Geometry check sheet. Reference: the model listing, model coordinates, mm. A direction names the side the tool comes from. Coordinates: 2 decimals unless noted, no trailing zeros. Write each loop counter-clockwise with the first axis right and the second up, starting at its lowest first coordinate (ties: lowest second). Pieces come first, ordered by that corner, then holes.
from build123d import *

# Parameters (mm, degrees)
SKETCH1_W                      = 65
SKETCH1_H                      = 100
BOSS_EXTRUDE1_DEPTH            = 5
SKETCH2_R                      = 3.5
BOSS_EXTRUDE2_DEPTH            = 3
F_3_6_3_6_DIAMETER_HOLE1_D     = 3.6
CBORE_FOR_M3_SHCS1_D           = 3.4
CBORE_FOR_M3_SHCS1_CBORE_D     = 6.5
CBORE_FOR_M3_SHCS1_CBORE_DEPTH = 3
SKETCH9_W                      = 100
SKETCH9_H                      = 5
BOSS_EXTRUDE3_DEPTH            = 50
CBORE_FOR_M3_SHCS2_D           = 3.4
CBORE_FOR_M3_SHCS2_CBORE_D     = 6.5
CBORE_FOR_M3_SHCS2_CBORE_DEPTH = 3
F_5_1_5_1_DIAMETER_HOLE1_D     = 5.1
CUT_EXTRUDE1_DEPTH             = 1
FILLET1_R                      = 1
FILLET2_R                      = 5
CHAMFER2_SIZE                  = 0.5


with BuildPart() as part:
    # Sketch1 → Boss-Extrude1 (new body)
    with BuildSketch(Plane(origin=(0, 0, 0), x_dir=(1, 0, 0), z_dir=(0, 1, 0))):
        with Locations((32.5, -50)):
            Rectangle(SKETCH1_W, SKETCH1_H)
    extrude(amount=BOSS_EXTRUDE1_DEPTH)

    # Sketch2 → Boss-Extrude2 (add)
    with BuildSketch(Plane(origin=(0, 5, 0), x_dir=(1, 0, 0), z_dir=(0, 1, 0))):
        with Locations(Location((8, -21, 0), (0, 0, 270))):
            Circle(SKETCH2_R)
        with Locations(Location((57, -21, 0), (0, 0, 270))):
            Circle(SKETCH2_R)
        with Locations(Location((57, -79, 0), (0, 0, 270))):
            Circle(SKETCH2_R)
        with Locations(Location((8, -79, 0), (0, 0, 270))):
            Circle(SKETCH2_R)
    extrude(amount=BOSS_EXTRUDE2_DEPTH)

    # Ø3.6 (3.6) Diameter Hole1 (through all)
    with Locations(Plane(origin=(0, 8, 0), x_dir=(1, 0, 0), z_dir=(0, 1, 0))):
        with Locations((8, -21), (57, -21), (57, -79), (8, -79)):
            Hole(F_3_6_3_6_DIAMETER_HOLE1_D / 2)

    # CBORE for M3 SHCS1 (through all)
    with Locations(Plane(origin=(0, 5, 0), x_dir=(1, 0, 0), z_dir=(0, 1, 0))):
        with Locations((17.5, -7.5), (47.5, -7.5)):
            CounterBoreHole(CBORE_FOR_M3_SHCS1_D / 2, CBORE_FOR_M3_SHCS1_CBORE_D / 2, CBORE_FOR_M3_SHCS1_CBORE_DEPTH)

    # Sketch9 → Boss-Extrude3 (add)
    with BuildSketch(Plane.ZY):
        with Locations((50, 2.5)):
            Rectangle(SKETCH9_W, SKETCH9_H)
    extrude(amount=BOSS_EXTRUDE3_DEPTH)

    # CBORE for M3 SHCS2 (through all)
    with Locations(Plane(origin=(0, 5, 0), x_dir=(1, 0, 0), z_dir=(0, 1, 0))):
        with Locations((-42.5, -45), (-12.5, -7.5), (-42.5, -7.5), (-12.5, -45)):
            CounterBoreHole(CBORE_FOR_M3_SHCS2_D / 2, CBORE_FOR_M3_SHCS2_CBORE_D / 2, CBORE_FOR_M3_SHCS2_CBORE_DEPTH)

    # Ø5.1 (5.1) Diameter Hole1 (through all)
    with Locations(Plane(origin=(0, 5, 0), x_dir=(1, 0, 0), z_dir=(0, 1, 0))):
        with Locations((-12.5, -26.25), (-12.5, -60), (-12.5, -90), (-42.5, -90), (-42.5, -60), (-42.5, -26.25)):
            Hole(F_5_1_5_1_DIAMETER_HOLE1_D / 2)

    # Sketch16 → Cut-Extrude1 (cut)
    with BuildSketch(Plane(origin=(0, 5, 0), x_dir=(1, 0, 0), z_dir=(0, 1, 0))):
        with BuildLine():
            Line((39.126262207, -50.847545166), (39.126262207, -49.597897606))
            add(Edge.make_bspline(
                [(39.126262207, -49.597897606), (38.887061603, -49.575713781), (38.426953933, -49.5330427), (37.765335099, -49.467029699), (37.16050318, -49.395654418), (36.608878249, -49.329176979), (36.103389832, -49.260432621), (35.637684233, -49.194155672), (35.207796553, -49.125451167), (34.693851603, -49.042468377), (34.106849427, -48.930569543), (33.65316464, -48.833024779), (33.43663372, -48.786469421)],
                knots=[0, 0, 0, 0, 1.253096053, 2.41035807, 3.468180285, 4.429891672, 5.308555075, 6.129167563, 6.883542428, 7.579384342, 8.844708592, 10, 10, 10, 10], degree=3))
            add(Edge.make_bspline(
                [(33.43663372, -48.786469421), (33.362346649, -48.767894411), (33.217288497, -48.731623541), (33.012809199, -48.653717957), (32.825678299, -48.562470211), (32.654731085, -48.453628715), (32.502165181, -48.313171441), (32.378215441, -48.129778401), (32.270782782, -47.910183348), (32.22072951, -47.746398482), (32.194209557, -47.659619598)],
                knots=[0, 0, 0, 0, 1.028706086, 2.008723763, 2.935244992, 3.824118955, 4.724963072, 5.700873389, 6.781843246, 8, 8, 8, 8], degree=3))
            add(Edge.make_bspline(
                [(32.194209557, -47.659619598), (32.184050249, -47.593155924), (32.163986257, -47.461894353), (32.185456965, -47.261992825), (32.24760698, -47.068817641), (32.345988654, -46.886281707), (32.470276431, -46.723283517), (32.612903387, -46.590894898), (32.770825068, -46.49396615), (32.885825633, -46.461994139), (32.943034973, -46.44608902)],
                knots=[0, 0, 0, 0, 1.027404461, 2.029059083, 3.048769739, 4.122307651, 5.19302046, 6.17728816, 7.093255398, 8, 8, 8, 8], degree=3))
            add(Edge.make_bspline(
                [(32.943034973, -46.44608902), (33.019790611, -46.432729059), (33.159183567, -46.408466548), (33.358775166, -46.415044291), (33.530189985, -46.45624418), (33.682659012, -46.516761006), (33.820245014, -46.588705021), (33.94106644, -46.670397622), (34.053969979, -46.753634053), (34.125488835, -46.811784665), (34.161381149, -46.840968018)],
                knots=[0, 0, 0, 0, 1.397360562, 2.537692669, 3.559369145, 4.550448304, 5.47954959, 6.34367758, 7.168761249, 8, 8, 8, 8], degree=3))
            add(Edge.make_bspline(
                [(34.161381149, -46.840968018), (34.171740761, -46.84988817), (34.20290871, -46.876725361), (34.270587507, -46.926391538), (34.365875235, -47.009106142), (34.490280901, -47.108420261), (34.623007569, -47.217425956), (34.758849499, -47.313547894), (34.885293124, -47.395630136), (35.04302611, -47.483660165), (35.248195948, -47.563686604), (35.419904702, -47.590557351), (35.50734066, -47.604240227)],
                knots=[0, 0, 0, 0, 0.26063328, 0.784141858, 1.599335041, 2.665418653, 3.819900223, 4.873162956, 5.836886495, 6.693141337, 8.316111744, 10, 10, 10, 10], degree=3))
            Line((35.50734066, -47.604240227), (39.126262207, -48.073760986))
            Line((39.126262207, -48.073760986), (39.126262207, -47.466995697))
            add(Edge.make_bspline(
                [(39.126262207, -47.466995697), (39.120615941, -47.395372643), (39.108842141, -47.246021633), (39.011762919, -47.038358034), (38.893301343, -46.84311371), (38.780591009, -46.744004371), (38.726567612, -46.696500092)],
                knots=[0, 0, 0, 0, 0.957298162, 1.996193101, 3.039551627, 4, 4, 4, 4], degree=3))
            Line((38.726567612, -46.696500092), (38.098132133, -46.282358704))
            Line((38.098132133, -46.282358704), (38.098132133, -45.608175049))
            add(Edge.make_bspline(
                [(38.098132133, -45.608175049), (38.265069197, -45.651305716), (38.590637549, -45.73542113), (39.059543061, -45.904315208), (39.510452961, -46.111726833), (39.782169404, -46.301225336), (39.9208358, -46.397933044)],
                knots=[0, 0, 0, 0, 1.033858386, 2.016278253, 2.987637474, 4, 4, 4, 4], degree=3))
            add(Edge.make_bspline(
                [(39.9208358, -46.397933044), (39.980466774, -46.441596233), (40.101066248, -46.529901979), (40.265647201, -46.68871056), (40.416093013, -46.870100588), (40.556417575, -47.068585687), (40.676744862, -47.287138148), (40.759698519, -47.527310442), (40.812591451, -47.784126696), (40.818378437, -47.961125766), (40.821352539, -48.052090797)],
                knots=[0, 0, 0, 0, 0.904302346, 1.828888262, 2.791608349, 3.786843382, 4.80268608, 5.834756118, 6.887217442, 8, 8, 8, 8], degree=3))
            Line((40.821352539, -48.052090797), (40.821352539, -54.430349731))
            Line((40.821352539, -54.430349731), (39.126262207, -54.430349731))
            Line((39.126262207, -54.430349731), (39.126262207, -52.369273987))
            add(Edge.make_bspline(
                [(39.126262207, -52.369273987), (38.824641017, -52.338588763), (38.212494456, -52.276312453), (37.278571929, -52.215269505), (36.316663871, -52.178581692), (35.66628914, -52.174105191), (35.336386948, -52.171834488)],
                knots=[0, 0, 0, 0, 0.958130554, 1.944546155, 2.957372268, 4, 4, 4, 4], degree=3))
            add(Edge.make_bspline(
                [(35.336386948, -52.171834488), (35.216918961, -52.176632011), (34.979958118, -52.18614774), (34.699390908, -52.267738632), (34.498680733, -52.345822532), (34.376377238, -52.399383952), (34.282754213, -52.45111856), (34.234840863, -52.489924695), (34.214352722, -52.506518517)],
                knots=[0, 0, 0, 0, 1.804721428, 3.579605919, 4.387653081, 5.067635593, 5.601313335, 6, 6, 6, 6], degree=3))
            add(Edge.make_bspline(
                [(34.214352722, -52.506518517), (34.158438507, -52.572803412), (34.054075473, -52.696523165), (33.974254217, -52.882970365), (33.965236632, -53.035635661), (33.99855982, -53.155268657), (34.063359986, -53.281985338), (34.125363446, -53.363077846), (34.158973351, -53.407035255)],
                knots=[0, 0, 0, 0, 1.530222605, 2.85613729, 3.495539136, 4.19786485, 5.023125643, 6, 6, 6, 6], degree=3))
            add(Edge.make_bspline(
                [(34.158973351, -53.407035255), (34.202678445, -53.453603851), (34.288209182, -53.54473845), (34.449483531, -53.638340717), (34.618180335, -53.696546772), (34.801341682, -53.734863252), (35.02056346, -53.757230953), (35.181594158, -53.781052837), (35.27378418, -53.794690857)],
                knots=[0, 0, 0, 0, 0.943448386, 1.846325613, 2.731669575, 3.584362821, 4.617048522, 6, 6, 6, 6], degree=3))
            Line((35.27378418, -53.794690857), (35.27378418, -54.543516273))
            add(Edge.make_bspline(
                [(35.27378418, -54.543516273), (35.145259799, -54.539686724), (34.899665229, -54.532368918), (34.549534649, -54.49381644), (34.23492324, -54.435411311), (33.95485327, -54.352646637), (33.704937688, -54.251951832), (33.47764334, -54.142729191), (33.274451352, -54.017945692), (33.089768771, -53.886609091), (32.927584898, -53.741089605), (32.786131125, -53.584968182), (32.654824603, -53.424803574), (32.58524624, -53.30689432), (32.550563774, -53.248120537)],
                knots=[0, 0, 0, 0, 1.463419428, 2.796417783, 4.006075808, 5.101867847, 6.114868065, 7.071137589, 7.969092879, 8.826327314, 9.648155468, 10.443549341, 11.224161887, 12, 12, 12, 12], degree=3))
            add(Edge.make_bspline(
                [(32.550563774, -53.248120537), (32.520790697, -53.193492864), (32.459254397, -53.080585998), (32.397200219, -52.890384649), (32.348206864, -52.6819503), (32.320086722, -52.457698844), (32.315640727, -52.227756787), (32.34661926, -52.004027153), (32.413206209, -51.79241002), (32.487069025, -51.66662071), (32.524077988, -51.603593979)],
                knots=[0, 0, 0, 0, 0.865492594, 1.788838003, 2.776551332, 3.847715376, 4.932865467, 5.972249091, 6.983995453, 8, 8, 8, 8], degree=3))
            add(Edge.make_bspline(
                [(32.524077988, -51.603593979), (32.599388708, -51.507318221), (32.75324726, -51.310628445), (33.055018494, -51.068656229), (33.409086865, -50.860800161), (33.672452045, -50.758731497), (33.809842529, -50.705485039)],
                knots=[0, 0, 0, 0, 0.918076197, 1.875614441, 2.891765566, 4, 4, 4, 4], degree=3))
            add(Edge.make_bspline(
                [(33.809842529, -50.705485039), (33.898631758, -50.682441773), (34.087470798, -50.633432807), (34.395240763, -50.584968257), (34.740993079, -50.551926433), (35.248657148, -50.532699083), (35.895954097, -50.531314455), (36.413618911, -50.570608952), (36.667899666, -50.589910698)],
                knots=[0, 0, 0, 0, 0.574329406, 1.22149743, 1.948877103, 2.749030755, 4.403100056, 6, 6, 6, 6], degree=3))
            Line((36.667899666, -50.589910698), (39.126262207, -50.847545166))
        make_face()
    extrude(amount=-CUT_EXTRUDE1_DEPTH, mode=Mode.SUBTRACT)

    # Fillet1
    fillet1_edges = [part.edges().sort_by_distance(p)[0] for p in [
        (8, 5, 17.5),
        (57, 5, 17.5),
        (57, 5, 75.5),
        (8, 5, 75.5),
    ]]
    fillet(fillet1_edges, radius=FILLET1_R)

    # Fillet2
    fillet2_edges = [part.edges().sort_by_distance(p)[0] for p in [
        (-50, 2.5, 0),
        (-50, 2.5, 100),
        (65, 2.5, 0),
        (65, 2.5, 100),
    ]]
    fillet(fillet2_edges, radius=FILLET2_R)

    # Chamfer2
    chamfer2_edges = [part.edges().sort_by_distance(p)[0] for p in [
        (8, 8, 17.5),
        (57, 8, 17.5),
        (57, 8, 75.5),
        (8, 8, 75.5),
    ]]
    chamfer(chamfer2_edges, length=CHAMFER2_SIZE)


solid = part.part
1. Sectioned sample at B-B, the plane z = 90. Record the boundary of the cut face in (x, y), and give its area (3 significant figures).
Computed values:
outline: (-50, 0) - (-45.05, 0) - (-45.05, 5) - (-50, 5) - close; (-39.95, 0) - (-15.05, 0) - (-15.05, 5) - (-39.95, 5) - close; (-9.95, 0) - (65, 0) - (65, 5) - (-9.95, 5) - close
area: 524 mm2
2. Sectioned sample at A-A, the plane x = 47.5. Record the boundary of the cut face in (y, z).
Computed values:
outline: (0, 0) - (5, 0) - (5, 4.25) - (2, 4.25) - (2, 5.8) - (0, 5.8) - close; (0, 9.2) - (2, 9.2) - (2, 10.75) - (5, 10.75) - (5, 100) - (0, 100) - close
3. Thickness scan on line 1 along Z through (x, y) = (-12.5, 4.15); line 2 along X through (y, z) = (0.7, 7.5); line 3 along Z through (x, y) = (-42.5, 1.2). Record the ranges inside material, lowest first.
Computed values:
line 1: z = 0 to 4.25, 10.75 to 23.7, 28.8 to 41.75, 48.25 to 57.45, 62.55 to 87.45, 92.55 to 100
line 2: x = -50 to -44.2, -40.8 to -14.2, -10.8 to 15.8, 19.2 to 45.8, 49.2 to 65
line 3: z = 0 to 5.8, 9.2 to 23.7, 28.8 to 43.3, 46.7 to 57.45, 62.55 to 87.45, 92.55 to 100
4. Gauge pin test, flat ends, axial feed: pin 1 Ø10.5 at (x, z) = (-12.5, 7.5) entering from +Y; pin 2 Ø5.5 at (x, z) = (17.5, 7.5) entering from +Y. Record the tip position at first contact, or that the pin passes through.
Computed values:
pin 1: stops at y = 5
pin 2: stops at y = 2
5. Sectioned sample at C-C, the plane x = -12.5. Give the number of separate pieces and of enclosed holes in the cut face, and give its area (3 significant figures).
Computed values:
separate pieces: 6
enclosed holes: 0
area: 371 mm2
6. Access from +Z, -Z, +X, -X, +Y, -Y to the whole of each face (thin tool, end or side, straight path). Record for faces 4 (the cylindrical face through (6.659, 6.74, 24.233)), 5 (the flat face through (57, 8, 23)).
Computed values:
face 4: +Y
face 5: +Z, -Z, +X, -X, +Y
7. Draft check along X on faces 1 (the cylindrical face through (57.234, 3.944, 19.215)), 2 (the cylindrical face through (64, 3, 98)), 3 (the flat face through (8, 0, 49)). Enter one of: released by +X, released by -X, zero draft, split by the parting line, or undercut.
Computed values:
face 1: undercut
face 2: released by +X
face 3: zero draft
